Source: CAD feature listing. Evaluate the final solid. Frame: model axes, mm. A direction names the side the tool comes from. Give positions to 0.01 mm unless a question says otherwise; leave off trailing zeros. Write each loop counter-clockwise with the first axis right and the second up, starting at its lowest first coordinate (ties: lowest second). Pieces come first, ordered by that corner, then holes.
```python
from build123d import *

# Parameters (mm, degrees)
SKETCH1_W           = 35.56
SKETCH1_H           = 12.7
BOSS_EXTRUDE1_DEPTH = 5.08
BOSS_EXTRUDE2_DEPTH = 5.08
SKETCH3_R           = 3.175
CUT_EXTRUDE1_DEPTH  = 36.56


with BuildPart() as part:
    # Sketch1 → Boss-Extrude1 (new body)
    with BuildSketch(Plane(origin=(0, 0, 0), x_dir=(1, 0, 0), z_dir=(0, 1, 0))):
        Rectangle(SKETCH1_W, SKETCH1_H)
    extrude(amount=BOSS_EXTRUDE1_DEPTH)

    # Sketch2 → Boss-Extrude2 (add)
    with BuildSketch(Plane(origin=(17.78, 0, 0), x_dir=(0, 0, -1), z_dir=(1, 0, 0))):
        with BuildLine():
            Line((-6.35, 5.08), (-3.062998127, 17.347257994))
            ThreePointArc((-3.062998127, 17.347257994), (0, 18.61599336), (3.062998127, 17.347257994))
            Line((3.062998127, 17.347257994), (6.35, 5.08))
            Line((6.35, 5.08), (-6.35, 5.08))
        make_face()
    boss_extrude2 = extrude(amount=-BOSS_EXTRUDE2_DEPTH)

    # Mirror1: Boss-Extrude2 across plane
    add(boss_extrude2.mirror(Plane(origin=(0, 0, 0), x_dir=(0, 0, 1), z_dir=(1, 0, 0))))

    # Sketch3 → Cut-Extrude1 (cut, through all)
    with BuildSketch(Plane(origin=(17.78, 0, 0), x_dir=(0, 0, -1), z_dir=(1, 0, 0))):
        with Locations((0, 12.7)):
            Circle(SKETCH3_R)
    extrude(amount=-CUT_EXTRUDE1_DEPTH, mode=Mode.SUBTRACT)


solid = part.part
```
1. Cut plane C-C, the plane y = 7.5. Return the cut outline in (x, z).
2. Contact query for flat-ended pins moving along their axis: P1, Ø10, axis at x = 11.5, y = 15.5, coming from the +Z side; P2, Ø4, axis at x = 6.5, z = 0.5, coming from the +Y side; P3, Ø3, axis at x = -14, z = -4, coming from the +Y side. Output: stop coordinate, or through.
3. Cut plane A-A, the plane z = 0. Return the cut outline in (x, y) (3 decimals).
4. Cut plane D-D, the plane y = 12.7. Return the cut outline in (x, z) (3 decimals).
5. Cut plane B-B, the plane x = -13.5. Return the cut outline in (y, z) (3 decimals), then the cut area to 3 significant figures.
6. Access query for faces 1 (the flat face through (-12.7, 9, 0)), 2 (the flat face through (0, 0, 0)). Directions: +Z, -Z, +X, -X, +Y, -Y. A direction counts if a zero-diameter tool reaches every point of the face in a straight line with its end or side. Return the directions, or none.
7. Line query: L1, parallel to Y at x = 15.4, z = 0 (3 decimals); L2, parallel to X at y = 8.5, z = -4.25; L3, parallel to Y at x = 8, z = -1.25. Output: solid intervals per line, ascending.
8. Mould query, pull axis X, two halves, no side actions, for faces 3 (the flat face through (17.78, 7, 0)), 4 (the flat face through (0, 5.08, 0)), 5 (the flat face through (12.7, 9, 0)), 6 (the flat face through (15.276, 11.299, -4.683)). Classes: +X half, -X half, draft (parallel to the pull), parting line (faces both ways), or undercut.
Response values:
1. outline: (-17.78, -5.7) - (-12.7, -5.7) - (-12.7, 5.7) - (-17.78, 5.7) - close; (12.7, -5.7) - (17.78, -5.7) - (17.78, 5.7) - (12.7, 5.7) - close
2. P1: stops at z = 4.86
2. P2: stops at y = 5.08
2. P3: stops at y = 17.82
3. outline: (-17.78, 0) - (17.78, 0) - (17.78, 9.525) - (12.7, 9.525) - (12.7, 5.08) - (-12.7, 5.08) - (-12.7, 9.525) - (-17.78, 9.525) - close; (-17.78, 15.875) - (-12.7, 15.875) - (-12.7, 18.616) - (-17.78, 18.616) - close; (12.7, 15.875) - (17.78, 15.875) - (17.78, 18.616) - (12.7, 18.616) - close
4. outline: (-17.78, -4.308) - (-12.7, -4.308) - (-12.7, -3.175) - (-17.78, -3.175) - close; (-17.78, 3.175) - (-12.7, 3.175) - (-12.7, 4.308) - (-17.78, 4.308) - close; (12.7, -4.308) - (17.78, -4.308) - (17.78, -3.175) - (12.7, -3.175) - close; (12.7, 3.175) - (17.78, 3.175) - (17.78, 4.308) - (12.7, 4.308) - close
5. outline: (0, -6.35) - (5.08, -6.35) - (17.347, -3.063) arc R4.332 ccw to (17.347, 3.063) - (5.08, 6.35) - (0, 6.35) - close; hole circle Ø6.35 at (12.7, 0)
5. area: 154 mm2
6. face 1: +Z, -Z, +Y
6. face 2: +Z, -Z, +X, -X, -Y
7. L1: y = 0 to 9.525, 15.875 to 18.616
7. L2: x = -17.78 to -12.7, 12.7 to 17.78
7. L3: y = 0 to 5.08
8. face 3: +X half
8. face 4: undercut
8. face 5: undercut
8. face 6: draft
